from build123d import *

# Parameters (mm, degrees)
F1_DEPTH = 25.4
F2_R     = 5.08


with BuildPart() as f1:
    # F0 (on Front) → F1 (new body)
    with BuildSketch(Plane.XZ):
        with BuildLine():
            Line((-35.6792770326, -26.9159432501), (35.6792770326, -26.9159432501))
            Line((35.6792770326, -26.9159432501), (35.6792770326, 26.9159432501))
            Line((35.6792770326, 26.9159432501), (-27.9675787613, 26.9159432501))
            ThreePointArc((-27.9675787613, 26.9159432501), (-30.2262828905, 21.462949108), (-35.6792770326, 19.2042449788))
            Line((-35.6792770326, 19.2042449788), (-35.6792770326, -26.9159432501))
        make_face()
    extrude(amount=F1_DEPTH)

    # F2
    f2_edges = [f1.edges().sort_by_distance(p)[0] for p in [
        (35.679277, -12.7, 26.915943),
        (-35.679277, -12.7, -26.915943),
        (35.679277, -12.7, -26.915943),
        (-35.679277, -12.7, 19.204245),
        (-27.967579, -12.7, 26.915943),
    ]]
    fillet(f2_edges, radius=F2_R)


solid = f1.part
Geometry check sheet. Reference: the model listing, model coordinates, mm. Coordinates: 2 decimals unless noted, no trailing zeros. Order: outer loops, then holes, each group sorted by start corner. A loop starts at its lowest first (then second) coordinate and runs counter-clockwise, first axis right, second up. Notation, with made-up numbers: (-9.5, -38) - (22.5, -38) arc R27 ccw to (22.5, -1) - close; hole circle Ø1 at (86, -30.75). An arc over 180 degrees is marked (long way). Answer in a Markdown table with one row per item. Add a question column.
1) Material ranges on line 1 along X through (y, z) = (-9, -23); line 2 along X through (y, z) = (-22, 17), recorded low to high. Write a range as [from, to].
2) Cross-section at A-A, the plane y = -19. Record the cut outline in (x, z), then the cut area to 3 significant figures.
3) Cross-section at B-B, the plane z = 23. Record the cut outline in (x, y), then the cut area to 3 significant figures.
Check result:
| question | item | result |
|---|---|---|
| 1 | line 1 | x = [-35.54, 35.54] |
| 1 | line 2 | x = [-35.34, 35.68] |
| 2 | outline | (-35.68, -21.84) arc R5.08 ccw to (-30.6, -26.92) - (30.6, -26.92) arc R5.08 ccw to (35.68, -21.84) - (35.68, 21.84) arc R5.08 ccw to (30.6, 26.92) - (-23.94, 26.92) arc R5.08 ccw to (-28.6, 23.85) arc R7.71 cw to (-32.62, 19.84) arc R5.08 ccw to (-35.68, 15.18) - close |
| 2 | area | 3,770 mm² |
| 3 | outline | (-29.04, -25.4) - (35.54, -25.4) - (35.54, 0) - (-29.04, 0) - close |
| 3 | area | 1,640 mm² |
